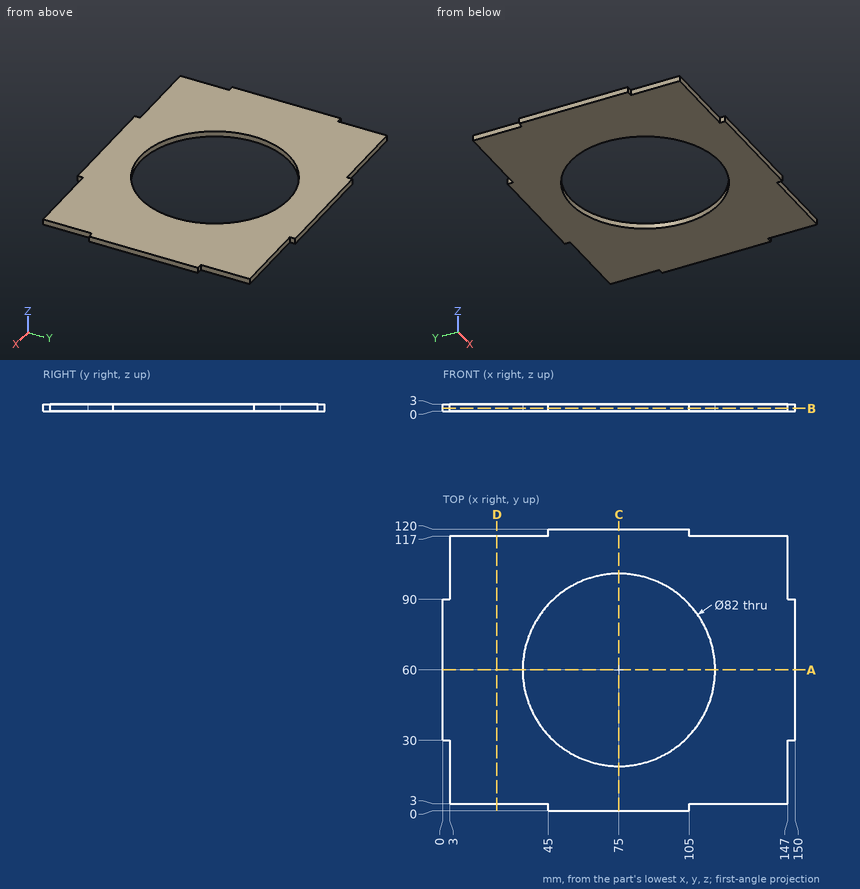
Source: three-view drawing plus pictorial views. Frame: mm from the lowest corner of the part. Coordinates: 2 decimals unless noted, no trailing zeros. Write each loop counter-clockwise with the first axis right and the second up, starting at its lowest first coordinate (ties: lowest second). Pieces come first, ordered by that corner, then holes. Notation, with made-up numbers: (66.25, -34.5) - (116.25, -34.5) arc R21 ccw to (116.25, -9.5) - close; hole circle Ø10 at (-19.5, 77.25). An arc over 180 degrees is marked (long way). Return JSON: item names as keys, results as strings.
Item 1: Section query C-C (x = 75). Output: boundary loops of the cut face in (y, z), and give its area (3 significant figures).
Completed:
{"outline": "(0, 0) - (19, 0) - (19, 3) - (0, 3) - close; (101, 0) - (120, 0) - (120, 3) - (101, 3) - close", "area": "114 mm2"}
Item 2: Section query A-A (y = 60). Output: boundary loops of the cut face in (x, z), and give its area (3 significant figures).
Completed:
{"outline": "(0, 0) - (34, 0) - (34, 3) - (0, 3) - close; (116, 0) - (150, 0) - (150, 3) - (116, 3) - close", "area": "204 mm2"}
Item 3: Line query: L1, parallel to Y at x = 75, z = 0.8; L2, parallel to X at y = 59, z = 2.4; L3, parallel to Y at x = 143, z = 0.45. Output: solid intervals per line, ascending.
Completed:
{"L1": "y = 0 to 19, 101 to 120", "L2": "x = 0 to 34.01, 115.99 to 150", "L3": "y = 3 to 117"}
Item 4: Section query D-D (x = 23). Output: boundary loops of the cut face in (y, z).
Completed:
{"outline": "(3, 0) - (117, 0) - (117, 3) - (3, 3) - close"}
Item 5: Pin query (flat end, axial travel): pin 1 Ø1.5 at (y, z) = (15, 2) entering from +X; pin 2 Ø1.5 at (x, z) = (2, 1) entering from +Y; pin 3 Ø1.5 at (x, z) = (26, 2) entering from -Y. Return the tip coordinate at first contact, or that it passes through.
Completed:
{"pin 1": "stops at x = 147", "pin 2": "stops at y = 90", "pin 3": "stops at y = 3"}
Item 6: Section query B-B (z = 1.1). Output: boundary loops of the cut face in (x, y).
Completed:
{"outline": "(0, 30) - (3, 30) - (3, 3) - (45, 3) - (45, 0) - (105, 0) - (105, 3) - (147, 3) - (147, 30) - (150, 30) - (150, 90) - (147, 90) - (147, 117) - (105, 117) - (105, 120) - (45, 120) - (45, 117) - (3, 117) - (3, 90) - (0, 90) - close; hole circle Ø82 at (75, 60)"}
